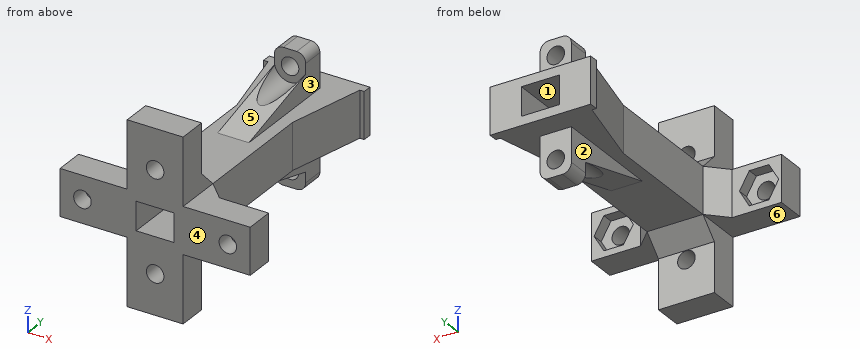
```python
from build123d import *
from OCP.BRepFilletAPI import BRepFilletAPI_MakeChamfer

# Parameters (mm, degrees)
SKETCH1_W           = 15.875
SKETCH1_H           = 13.208
BOSS_EXTRUDE1_DEPTH = 73.533
SHELL1_T            = -2.54
SKETCH3_W           = 8.89
SKETCH3_H           = 6.35
BOSS_EXTRUDE2_DEPTH = 12.319
SKETCH4_W           = 8.89
SKETCH4_H           = 6.35
BOSS_EXTRUDE3_DEPTH = 12.319
SKETCH5_W           = 13.208
SKETCH5_H           = 8.255
BOSS_EXTRUDE4_DEPTH = 19.05
SKETCH6_W           = 15.875
SKETCH6_H           = 8.255
BOSS_EXTRUDE5_DEPTH = 19.05
SKETCH7_W           = 13.208
SKETCH7_H           = 8.255
BOSS_EXTRUDE6_DEPTH = 19.05
SKETCH8_W           = 15.875
SKETCH8_H           = 8.255
BOSS_EXTRUDE7_DEPTH = 19.05
SKETCH9_R           = 2.4892
CUT_EXTRUDE1_DEPTH  = 83.847766424
CUT_EXTRUDE2_REACH  = 84.848
SKETCH11_R          = 2.4892
FILLET3_R           = 2.54
CHAMFER2_SIZE       = 25.4
CHAMFER2_SIZE_2     = 6.805909488
SKETCH12_R          = 4.445
CUT_EXTRUDE3_DEPTH  = 52.07
SKETCH13_W          = 28.575
SKETCH13_H          = 13.208
SKETCH13_W_2        = 10.795
SKETCH13_H_2        = 8.128
BOSS_EXTRUDE8_DEPTH = 2.54
CHAMFER3_SIZE       = 5.08
CHAMFER3_SIZE2      = 22.003897441
CHAMFER4_SIZE       = 5.08
CHAMFER5_SIZE       = 5.08
CUT_EXTRUDE4_DEPTH  = 3.175
CUT_EXTRUDE5_DEPTH  = 3.175


# Some blends are built 0.0001 mm under size
with BuildPart() as part:
    # Sketch1 → Boss-Extrude1 (new body)
    with BuildSketch(Plane(origin=(0, 0, 0), x_dir=(1, 0, 0), z_dir=(0, 1, 0))):
        with Locations((0, 1.3335)):
            Rectangle(SKETCH1_W, SKETCH1_H)
    extrude(amount=BOSS_EXTRUDE1_DEPTH)

    # Shell1
    shell1_openings = [part.faces().sort_by_distance(p)[0] for p in [
        (0, 73.533, -1.3335),
        (0, 0, -1.3335),
    ]]
    offset(amount=SHELL1_T, openings=shell1_openings, kind=Kind.INTERSECTION)

    # Sketch3 → Boss-Extrude2 (add)
    with BuildSketch(Plane(origin=(0, 0, -7.9375), x_dir=(-1, 0, 0), z_dir=(0, 0, -1))):
        with Locations((0, 63.5)):
            Rectangle(SKETCH3_W, SKETCH3_H)
    extrude(amount=BOSS_EXTRUDE2_DEPTH)

    # Sketch4 → Boss-Extrude3 (add)
    with BuildSketch(Plane.XY.offset(5.2705)):
        with Locations((0, 63.5)):
            Rectangle(SKETCH4_W, SKETCH4_H)
    extrude(amount=BOSS_EXTRUDE3_DEPTH)

    # Sketch5 → Boss-Extrude4 (add)
    with BuildSketch(Plane.ZY.offset(7.9375)):
        with Locations((-1.3335, 4.1275)):
            Rectangle(SKETCH5_W, SKETCH5_H)
    extrude(amount=BOSS_EXTRUDE4_DEPTH)

    # Sketch6 → Boss-Extrude5 (add)
    with BuildSketch(Plane(origin=(0, 0, -7.9375), x_dir=(-1, 0, 0), z_dir=(0, 0, -1))):
        with Locations((0, 4.1275)):
            Rectangle(SKETCH6_W, SKETCH6_H)
    extrude(amount=BOSS_EXTRUDE5_DEPTH)

    # Sketch7 → Boss-Extrude6 (add)
    with BuildSketch(Plane(origin=(7.9375, 0, 0), x_dir=(0, 0, -1), z_dir=(1, 0, 0))):
        with Locations((1.3335, 4.1275)):
            Rectangle(SKETCH7_W, SKETCH7_H)
    extrude(amount=BOSS_EXTRUDE6_DEPTH)

    # Sketch8 → Boss-Extrude7 (add)
    with BuildSketch(Plane.XY.offset(5.2705)):
        with Locations((0, 4.1275)):
            Rectangle(SKETCH8_W, SKETCH8_H)
    extrude(amount=BOSS_EXTRUDE7_DEPTH)

    # Sketch9 → Cut-Extrude1 (cut, through all)
    with BuildSketch(Plane(origin=(0, 73.533, 0), x_dir=(1, 0, 0), z_dir=(0, 1, 0))):
        with Locations((0, 15.621)):
            Circle(SKETCH9_R)
        with Locations((0, -12.954)):
            Circle(SKETCH9_R)
    extrude(amount=-CUT_EXTRUDE1_DEPTH, mode=Mode.SUBTRACT)

    # Sketch11 → Cut-Extrude2 (cut, up to next)
    with BuildSketch(Plane(origin=(0, 0, 0), x_dir=(-1, 0, 0), z_dir=(0, -1, 0)), mode=Mode.PRIVATE) as cut_extrude2_sk1:
        with Locations(Location((20.6375, 1.3335, 0), (0, 0, 90))):
            Circle(SKETCH11_R)
    cut_extrude2_tool1 = extrude(cut_extrude2_sk1.sketch, amount=-CUT_EXTRUDE2_REACH, mode=Mode.PRIVATE) & part.part
    # Sketch11 → Cut-Extrude2 (cut, up to next)
    with BuildSketch(Plane(origin=(0, 0, 0), x_dir=(-1, 0, 0), z_dir=(0, -1, 0)), mode=Mode.PRIVATE) as cut_extrude2_sk2:
        with Locations(Location((-20.6375, 1.3335, 0), (0, 0, 90))):
            Circle(SKETCH11_R)
    cut_extrude2_tool2 = extrude(cut_extrude2_sk2.sketch, amount=-CUT_EXTRUDE2_REACH, mode=Mode.PRIVATE) & part.part
    add(cut_extrude2_tool1.solids().sort_by_distance((-20.6375, 0, -1.3335))[0], mode=Mode.SUBTRACT)
    add(cut_extrude2_tool2.solids().sort_by_distance((20.6375, 0, -1.3335))[0], mode=Mode.SUBTRACT)

    # Fillet3
    fillet3_edges = [part.edges().sort_by_distance(p)[0] for p in [
        (4.445, 63.5, -20.2565),
        (-4.445, 63.5, -20.2565),
        (4.445, 63.5, 17.5895),
        (-4.445, 63.5, 17.5895),
    ]]
    fillet(fillet3_edges, radius=FILLET3_R)

    # Chamfer2
    # the kernel refuses this chamfer: 25.4, 6.805909488 mm, written as the material it adds along each edge
    with BuildSketch(Plane(origin=(-4.445, 60.325, -7.9375), x_dir=(0, -0.9999503267608393, 0.00996714657715642), z_dir=(1, 0, 0))) as chamfer2_piece_1_section:
        Polygon((CHAMFER2_SIZE * 0.999950326761, CHAMFER2_SIZE * 0.00996714657716), (-CHAMFER2_SIZE_2 * 0.00996714657679, CHAMFER2_SIZE_2 * 0.999950326724), (0, 0), align=None)
    chamfer2_piece_1 = extrude(amount=8.89, mode=Mode.PRIVATE)
    chamfer2_piece_1 = chamfer2_piece_1 - Plane(origin=(0, 51.301210878, -15.621), x_dir=(1, 0, 0), z_dir=(0, 1, 0)) * Cylinder(2.4892, 120, mode=Mode.PRIVATE)
    add(chamfer2_piece_1)
    with BuildSketch(Plane(origin=(4.445, 60.325, 5.2705), x_dir=(0, -0.9999503267608393, -0.00996714657715642), z_dir=(-1, 0, 0))) as chamfer2_piece_2_section:
        Polygon((CHAMFER2_SIZE * 0.999950326761, CHAMFER2_SIZE * 0.00996714657716), (-CHAMFER2_SIZE_2 * 0.00996714657679, CHAMFER2_SIZE_2 * 0.999950326724), (0, 0), align=None)
    chamfer2_piece_2 = extrude(amount=8.89, mode=Mode.PRIVATE)
    chamfer2_piece_2 = chamfer2_piece_2 - Plane(origin=(0, 51.301210878, 12.954), x_dir=(1, 0, 0), z_dir=(0, 1, 0)) * Cylinder(2.4892, 120, mode=Mode.PRIVATE)
    add(chamfer2_piece_2)

    # Sketch12 → Cut-Extrude3 (cut)
    with BuildSketch(Plane.XZ.offset(-60.325)):
        with Locations((0, -15.621)):
            Circle(SKETCH12_R)
        with Locations((0, 12.954)):
            Circle(SKETCH12_R)
    extrude(amount=CUT_EXTRUDE3_DEPTH, mode=Mode.SUBTRACT)

    # Sketch13 → Boss-Extrude8 (add)
    with BuildSketch(Plane(origin=(0, 73.533, 0), x_dir=(1, 0, 0), z_dir=(0, 1, 0))):
        with Locations((0, 1.3335)):
            Rectangle(SKETCH13_W, SKETCH13_H)
        with Locations((0, 1.3335)):
            Rectangle(SKETCH13_W_2, SKETCH13_H_2, mode=Mode.SUBTRACT)
    extrude(amount=-BOSS_EXTRUDE8_DEPTH)

    # Chamfer3: one chamfer whose edges measure the first distance from different faces: ONE call of the kernel's chamfer builder (chamfer() names one face for all edges)
    chamfer3_edges_1 = [part.edges().sort_by_distance(p)[0] for p in [
        (7.9375, 70.993, -1.3335),
    ]]
    chamfer3_side_1 = [part.faces().sort_by_distance(p)[0] for p in [
        (11.1125, 70.993, -1.3335),
    ]]
    chamfer3_edges_2 = [part.edges().sort_by_distance(p)[0] for p in [
        (-7.9375, 70.993, -1.3335),
    ]]
    chamfer3_side_2 = [part.faces().sort_by_distance(p)[0] for p in [
        (-11.1125, 70.993, -1.3335),
    ]]
    chamfer3 = BRepFilletAPI_MakeChamfer(part.part.solid().wrapped)
    for e in chamfer3_edges_1:
        chamfer3.Add(CHAMFER3_SIZE, CHAMFER3_SIZE2, e.wrapped, chamfer3_side_1[0].wrapped)  # the first distance lies on this face
    for e in chamfer3_edges_2:
        chamfer3.Add(CHAMFER3_SIZE, CHAMFER3_SIZE2, e.wrapped, chamfer3_side_2[0].wrapped)  # the first distance lies on this face
    add(Compound.cast(chamfer3.Shape()), mode=Mode.REPLACE)

    # Chamfer4
    # the kernel refuses this chamfer: 5.08 mm, written as the material it adds along each edge
    with BuildSketch(Plane(origin=(-7.9375, 8.255, -7.9375), x_dir=(0, 0.9996219169112968, 0.027495876610586438), z_dir=(1, 0, 0)), Plane(origin=(7.9375, 8.255, 5.2705), x_dir=(0, 0.9996219169112968, -0.027495876610586438), z_dir=(-1, 0, 0))) as chamfer4_piece_1:
        Polygon((CHAMFER4_SIZE * 0.999621916911, -CHAMFER4_SIZE * 0.0274958766106), (-CHAMFER4_SIZE * 0.0274958766106, -CHAMFER4_SIZE * 0.999621916911), (0, 0), align=None)
    extrude(amount=15.875)

    # Chamfer5
    chamfer5_edges = [part.edges().sort_by_distance(p)[0] for p in [
        (-7.9375, 8.255, -1.3335),
        (7.9375, 8.255, -1.3335),
    ]]
    chamfer(chamfer5_edges, length=CHAMFER5_SIZE - 0.0001)  # a hair under: the kernel refuses the full size

    # Sketch14 → Cut-Extrude4 (cut)
    with BuildSketch(Plane(origin=(0, 8.255, 0), x_dir=(1, 0, 0), z_dir=(0, 1, 0))):
        Polygon((-26.210084798, 1.3335), (-23.423792399, -3.4925), (-17.851207601, -3.4925), (-15.064915202, 1.3335), (-17.851207601, 6.1595), (-23.423792399, 6.1595), align=None)
    extrude(amount=-CUT_EXTRUDE4_DEPTH, mode=Mode.SUBTRACT)

    # Sketch15 → Cut-Extrude5 (cut)
    with BuildSketch(Plane(origin=(0, 8.255, 0), x_dir=(1, 0, 0), z_dir=(0, 1, 0))):
        Polygon((15.064915202, 1.3335), (17.851207601, -3.4925), (23.423792399, -3.4925), (26.210084798, 1.3335), (23.423792399, 6.1595), (17.851207601, 6.1595), align=None)
    extrude(amount=-CUT_EXTRUDE5_DEPTH, mode=Mode.SUBTRACT)


solid = part.part
```
Build history of the part. All positions in model axes, mm. Face numbers are marked on the shaded views. A direction names the side the tool comes from. Give positions to 0.01 mm unless a question says otherwise; leave off trailing zeros. Order: outer loops, then holes, each group sorted by start corner. A loop starts at its lowest first (then second) coordinate and runs counter-clockwise, first axis right, second up. Notation, with made-up numbers: M 43,-12.75 L 55,-12.75 A21 cw 55,9.25 Z; hole C 6.25,63.5 d7. An arc over 180 degrees is marked long. Write item = value, one per line. Start each with the question number.
(1) Slice it at C-C on z = -16.5. Write the cut outline in (x, y) (1 decimal), plus the area to 3 significant figures.
(2) Slice it at B-B on x = 9. Write the cut outline in (y, z).
(3) Slice it at A-A on y = 25. Write the cut outline in (x, z).
(4) Slice it at D-D on x = -19. Write the cut outline in (y, z) (1 decimal), plus the area to 3 significant figures.
(5) Probe L1, parallel to Z at x = 0, y = 3.25; L2, parallel to X at y = 36, z = 2.5; L3, parallel to Z at x = 0, y = 29. List the from-to ranges inside material, lowest first. Write a range as [from, to].
(6) Pin check, flat tips, straight feed: pin 1 Ø12 at (x, y) = (2, 21) entering from -Z; pin 2 Ø1 at (x, z) = (-10, -18.5) entering from -Y; pin 3 Ø3 at (x, z) = (22, 1) entering from +Y; pin 4 Ø3 at (x, y) = (0.5, 42.5) entering from +Z. Stop position of each tip, or through.
(7) Which spindle directions (+Z, -Z, +X, -X, +Y, -Y) get a long thin tool onto all of the face, cutting with end or side? Do the marked faces 1, 2 and 3. Say none if no direction does.
(8) Two-plate mould, pull along Y, no slides. Class the marked faces 4, 5 and 6: released by +Y, released by -Y, zero draft, split by the parting line, or undercut.
Responses:
q1.outline = M -7.9,0 L -2.3,0 L -2.3,8.3 L -7.9,8.3 Z; M -4.4,60.3 L -2.3,60.3 L -2.3,66.7 L -4.4,66.7 Z; M 2.3,0 L 7.9,0 L 7.9,8.3 L 2.3,8.3 Z; M 2.3,60.3 L 4.4,60.3 L 4.4,66.7 L 2.3,66.7 Z
q1.area = 119 mm2
q2.outline = M 0,-7.94 L 12.27,-7.94 L 12.27,5.27 L 0,5.27 Z; M 53.59,-7.94 L 73.53,-7.94 L 73.53,5.27 L 53.59,5.27 Z
q3.outline = M -7.94,-7.94 L 7.94,-7.94 L 7.94,5.27 L -7.94,5.27 Z; hole M -5.4,-5.4 L 5.4,-5.4 L 5.4,2.73 L -5.4,2.73 Z
q4.outline = M 0,-7.9 L 8.3,-7.9 L 8.3,-6.2 L 5.1,-6.2 L 5.1,-3.2 L 0,-3.2 Z; M 0,0.5 L 5.1,0.5 L 5.1,3.5 L 8.3,3.5 L 8.3,5.3 L 0,5.3 Z
q4.area = 59.3 mm2
q5.L1 = [-26.99, -18.11], [-13.13, -5.4], [2.73, 10.46], [15.44, 24.32]
q5.L2 = [-7.94, -5.4], [5.4, 7.94]
q5.L3 = [-7.94, -5.4], [2.73, 5.27]
q6.pin_1 = -7.94
q6.pin_2 = through
q6.pin_3 = 5.08
q6.pin_4 = 7.7
q7.face_1 = +Y, -Y
q7.face_2 = -Z, -X, +Y
q7.face_3 = +Z, +X, +Y
q8.face_4 = released by -Y
q8.face_5 = undercut
q8.face_6 = zero draft
